Could you check a few things on this drawing? It's one solid part, dimensions in mm from its lowest x, y, z. Round coordinates to 2 decimals unless told otherwise and drop trailing zeros. Loops run counter-clockwise (first coordinate to the right, second up) from the corner with the lowest first, then second, coordinate; pieces in that order, holes last. Notation, with made-up numbers: (-5, 54.25) -> (35, 54.25) arc R20 cw to (35, 90.25) -> close; hole circle Ø9 at (-30.75, 18.5). An arc over 180 degrees is marked (long way). Put each result on its own line as item: value. Start each with the question number.
1. Imagine slicing it at A-A, the plane x = 182. Please give me the cut outline in (y, z) (1 decimal).
2. Imagine slicing it at B-B, the plane z = 663. Count the separate pieces of the cut face and the enclosed holes in it, and give its area (3 significant figures).
3. Imagine slicing it at D-D, the plane x = 964. Please give me the cut outline in (y, z) (1 decimal).
4. I'm going to push a flat-ended pin straight in: P1, Ø4, axis at y = 6, z = 505, coming from the -X side. Where does the tip first touch, or does it pass through?
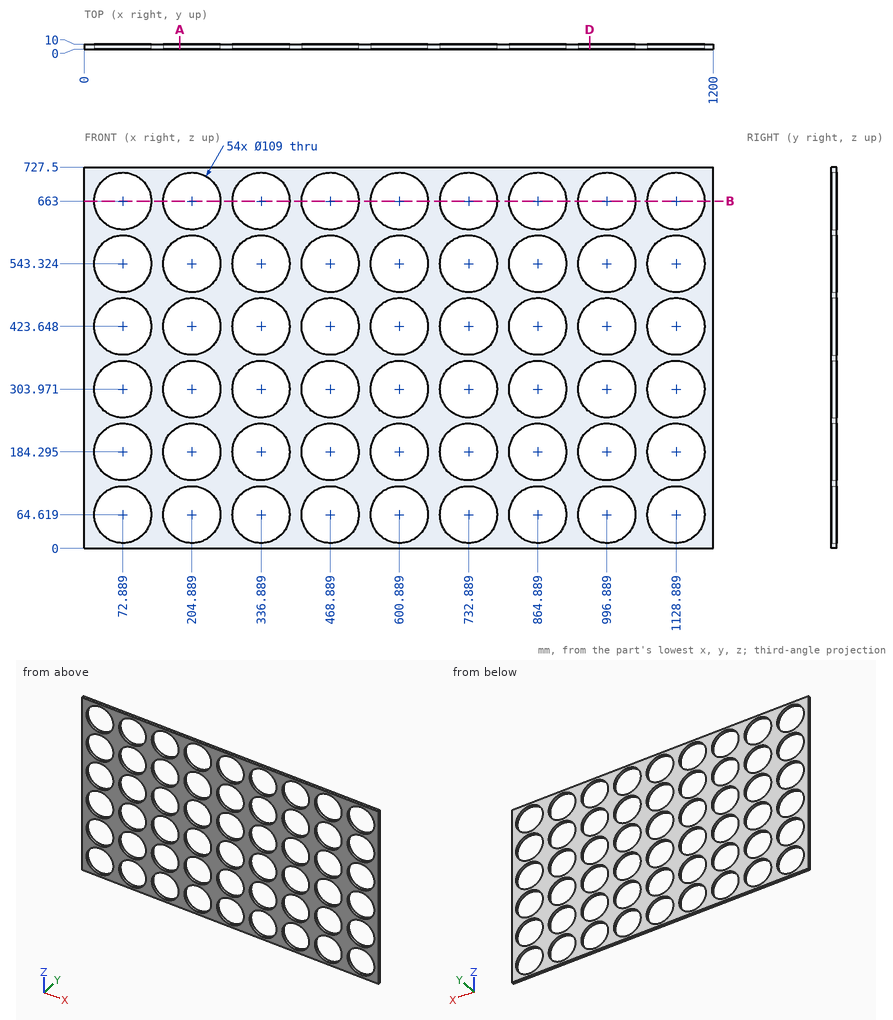
Entries:
1. outline: (0, 0) -> (10, 0) -> (10, 15.2) -> (0, 15.2) -> close; (0, 114.1) -> (10, 114.1) -> (10, 134.8) -> (0, 134.8) -> close; (0, 233.8) -> (10, 233.8) -> (10, 254.5) -> (0, 254.5) -> close; (0, 353.4) -> (10, 353.4) -> (10, 374.2) -> (0, 374.2) -> close; (0, 473.1) -> (10, 473.1) -> (10, 493.9) -> (0, 493.9) -> close; (0, 592.8) -> (10, 592.8) -> (10, 613.5) -> (0, 613.5) -> close; (0, 712.5) -> (10, 712.5) -> (10, 727.5) -> (0, 727.5) -> close
2. separate pieces: 10
2. enclosed holes: 0
2. area: 2,190 mm^2
3. outline: (0, 0) -> (10, 0) -> (10, 21.2) -> (0, 21.2) -> close; (0, 108.1) -> (10, 108.1) -> (10, 140.8) -> (0, 140.8) -> close; (0, 227.8) -> (10, 227.8) -> (10, 260.5) -> (0, 260.5) -> close; (0, 347.4) -> (10, 347.4) -> (10, 380.2) -> (0, 380.2) -> close; (0, 467.1) -> (10, 467.1) -> (10, 499.9) -> (0, 499.9) -> close; (0, 586.8) -> (10, 586.8) -> (10, 619.5) -> (0, 619.5) -> close; (0, 706.5) -> (10, 706.5) -> (10, 727.5) -> (0, 727.5) -> close
4. P1: x = 0
